Here's how the part is built. I have some questions about the finished solid (model axes, mm). Face numbers are marked on the shaded views. A direction names the side the tool comes from. Round coordinates to 2 decimals unless told otherwise and drop trailing zeros. Loops run counter-clockwise (first coordinate to the right, second up) from the corner with the lowest first, then second, coordinate; pieces in that order, holes last. Notation, with made-up numbers: M 67,2 L 116,2 A14 cw 116,11 Z; hole C 22.25,52 d1. An arc over 180 degrees is marked long. Put each result on its own line as item: value. Start each with the question number.
Autodesk Inventor part; units mm, degrees
ref_plane "YZ Plane" through (0, 0, 0) normal (1, 0, 0) x (0, 1, 0)
ref_plane "XZ Plane" through (0, 0, 0) normal (0, 1, 0) x (-1, 0, 0)
ref_plane "XY Plane" through (0, 0, 0) normal (0, 0, 1) x (1, 0, 0)
sketch "Sketch1" plane through (0, 0, 0) normal (0, 0, 1) x (1, 0, 0)
  circle A0 centre (0, 0) radius 2.4
  circle A1 centre (0, 0) radius 6
  dimension "d0" = 4.8
  dimension "d1" = 12
extrude "Extrusion1" add sketch "Sketch1" along normal blind 4 contours A0 | A1
extrude "Extrusion2" add sketch "Sketch1" against normal blind 11 contours A0
fillet "Fillet1" radius 1 1 edges at (-2.4, 0, 0)
fillet "Fillet2" radius 3 1 edges at (-6, 0, 4)
sketch "Sketch2" plane through (0, 0, 4) normal (0, 0, 1) x (1, 0, 0)
  line L0 (2.2, 0) -> (1.1, -1.9053)
  line L1 (1.1, -1.9053) -> (-1.1, -1.9053)
  line L2 (-1.1, -1.9053) -> (-2.2, 0)
  line L3 (-2.2, 0) -> (-1.1, 1.9053)
  line L4 (-1.1, 1.9053) -> (1.1, 1.9053)
  line L5 (1.1, 1.9053) -> (2.2, 0)
  point P0 (0, 0)
  point P1 (0, 0)
  dimension "d8" = 4.4
extrude "Extrusion3" cut sketch "Sketch2" against normal blind 3
thread "Thread1"
properties part number "SkaterInsertScrew" material "Stainless Steel"
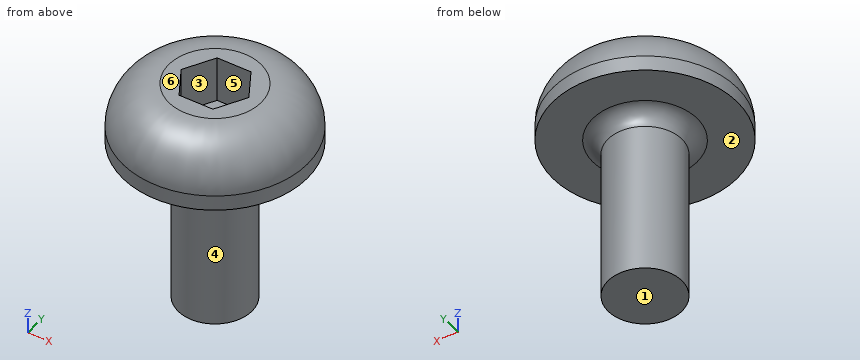
1) If I drill on probe 1 along X at (y, z) = (5.5, 0.5); probe 2 along Z at (x, y) = (0, 0.25); probe 3 along X at (y, z) = (1, 1.25), over which ranges is the centre line in solid material (lowest first)? Write a range as from..to.
2) Suppose I cut it at A-A (z = -6.5). Write out the boundary of the cut face in (x, y), plus the area to 3 significant figures.
3) If we mould it in two halves opening along Y, with no side actions, what happens to the marked faces 4, 5 and 6? For each: pulls with the +Y half, pulls with the -Y half, needs draft (parallel to the pull), parting line crosses it, or undercut.
4) I'm going to push flat-ended pins straight in: P1, Ø1.5, axis at x = -4, y = -2, coming from the -Z side; P2, Ø0.7, axis at x = 0, z = 3, coming from the +Y side; P3, Ø2.5, axis at x = 0.5, z = 3, coming from the -Y side. Where does each tip first touch, or does it pass through?
5) On a 3-axis mill with a long thin cutter (end or side, diameter ignored), from which of +Z, -Z, +X, -X, +Y, -Y can I reach the whole of each face in a straight line? I mean the marked faces 1, 2 and 3. Say none if no direction works.
Results are:
1. probe 1: -2.4..2.4
1. probe 2: -11..1
1. probe 3: -5.91..-1.62, 1.62..5.91
2. outline: C 0,0 d4.8
2. area: 18.1 mm²
3. face 4: parting line crosses it
3. face 5: undercut
3. face 6: needs draft
4. P1: z = 0
4. P2: y = 5.51
4. P3: y = -5.89
5. face 1: -Z, +X, -X, +Y, -Y
5. face 2: -Z
5. face 3: +Z
